Read the model definition and answer for the solid it produces. Units are mm, in the model's axes. A direction names the side the tool comes from. Round coordinates to 2 decimals unless told otherwise and drop trailing zeros. Order: outer loops, then holes, each group sorted by start corner. A loop starts at its lowest first (then second) coordinate and runs counter-clockwise, first axis right, second up. Notation, with made-up numbers: (30, -13.75) - (59, -13.75) arc R16 cw to (59, -6.75) - close; hole circle Ø9 at (22.25, 45.25). An arc over 180 degrees is marked (long way). Answer as a JSON object with one key per item and string values. Group by question number.
Q1. Consider line 1 (Z direction, x = -11, y = 92); line 2 (X direction, y = 104, z = -68.8); line 3 (Z direction, x = 11.5, y = 49). Determine where each line is inside the solid, lowest interval first.
Q2. The mould has two halves that part along Z. Classify faces 4 (the flat face through (-13, -9, 2)), 5 (the flat face through (-19, 52, -40)), 6 (the cylindrical face through (-14.096, -10.369, 3.014)): pulls with the +Z half, pulls with the -Z half, needs draft (parallel to the pull), parting line crosses it, or undercut.
Q3. A cutting plane is placed at D-D on z = -14.5. Determine the outline of the cut face in (x, y).
Q4. Given pin 1 Ø13 at (x, y) = (4.17, 91.16) entering from +Z; pin 2 Ø5 at (x, y) = (-10.92, 111.94) entering from -Z; pin 3 Ø6 at (y, z) = (31, -56) entering from +X; pin 4 Ø2 at (x, z) = (-2.5, -46) entering from -Y, each flat-ended and moving along its own axis, determine where each tip first touches the part or whether it passes through.
Q5. A cutting plane is placed at C-C on y = 28.5. Determine the outline of the cut face in (x, z), and give its area (3 significant figures).
Q6. A cutting plane is placed at A-A on z = -33. Determine the outline of the cut face in (x, y).
Q7. A cutting plane is placed at B-B on y = 0. Determine the outline of the cut face in (x, z).
Q8. A tool of negligible diameter and unlimited length cuts with its end or side. For faces 1 (the flat face through (0, 92, -68)), 2 (the flat face through (0, 12, 0)), 3 (the cylindrical face through (3.305, 120.744, -71.014)), from which of +Z, -Z, +X, -X, +Y, -Y can it reach the whole face along a straight path? Write none if from no direction.
```python
from build123d import *

# Parameters (mm, degrees)
BOSS_EXTRUDE2_DEPTH       = 4
BOSS_EXTRUDE3_START       = 68
BOSS_EXTRUDE3_DEPTH       = 68
BOSS_EXTRUDE4_START       = 4
BOSS_EXTRUDE4_DEPTH       = 4
BOSS_EXTRUDE5_START       = -4
BOSS_EXTRUDE5_DEPTH       = 4
CUT_EXTRUDE1_REACH        = 144.941
CUT_EXTRUDE2_DEPTH        = 143.940547082
BOSS_EXTRUDE7_DEPTH       = 10
BOSS_EXTRUDE7_DEPTH_BACK  = 10
SKETCH10_R                = 2
CUT_EXTRUDE3_DEPTH        = 4
SKETCH11_R                = 18
SKETCH11_R_2              = 16
BOSS_EXTRUDE8_DEPTH       = 4
MIRROR6_COPY_1_SKETCH_R   = 2
MIRROR6_COPY_1_DEPTH      = 4
MIRROR6_COPY_2_SKETCH_R   = 18
MIRROR6_COPY_2_SKETCH_R_2 = 16
MIRROR6_COPY_2_DEPTH      = 4
SKETCH12_R                = 4.000160783
SKETCH12_R_2              = 2
CUT_EXTRUDE5_DEPTH        = 2
MIRROR8_COPY_1_SKETCH_R   = 4.000160783
MIRROR8_COPY_1_SKETCH_R_2 = 2
MIRROR8_COPY_1_DEPTH      = 2
SKETCH13_W                = 4
SKETCH13_H                = 5
BOSS_EXTRUDE9_DEPTH       = 6
SKETCH14_W                = 20
SKETCH14_H                = 5
BOSS_EXTRUDE10_DEPTH      = 4
FILLET1_R                 = 5


with BuildPart() as part:
    # Sketch2 → Boss-Extrude2 (new body)
    with BuildSketch(Plane.XY):
        with BuildLine():
            Line((-16, 0), (-16, 30))
            ThreePointArc((-16, 30), (0, 46), (16, 30))
            Line((16, 30), (16, 0))
            ThreePointArc((16, 0), (0, -16), (-16, 0))
        make_face()
    extrude(amount=BOSS_EXTRUDE2_DEPTH)

    # Sketch3 → Boss-Extrude3 (add)
    with BuildSketch(Plane(origin=(0, 0, 0), x_dir=(-1, 0, 0), z_dir=(0, 0, -1)).offset(BOSS_EXTRUDE3_START)):
        with BuildLine():
            Line((-16, 30), (-16, 26))
            Line((-16, 26), (-12, 30))
            ThreePointArc((-12, 30), (0, 42), (12, 30))
            Line((12, 30), (16, 26))
            Line((16, 26), (16, 30))
            ThreePointArc((16, 30), (0, 46), (-16, 30))
        make_face()
    boss_extrude3 = extrude(amount=-BOSS_EXTRUDE3_DEPTH)

    # Sketch4 → Boss-Extrude4 (add)
    with BuildSketch(Plane(origin=(0, 0, -68), x_dir=(-1, 0, 0), z_dir=(0, 0, -1)).offset(BOSS_EXTRUDE4_START)):
        with BuildLine():
            Line((-16, 30), (-16, 0))
            ThreePointArc((-16, 0), (0, -16), (16, 0))
            Line((16, 0), (16, 30))
            ThreePointArc((16, 30), (0, 46), (-16, 30))
        make_face()
    boss_extrude4 = extrude(amount=-BOSS_EXTRUDE4_DEPTH)

    # Sketch5 → Boss-Extrude5 (add)
    with BuildSketch(Plane.XY.offset(4).offset(BOSS_EXTRUDE5_START)):
        with BuildLine():
            Line((-16, 120), (-16, 30))
            ThreePointArc((-16, 30), (0, 46), (16, 30))
            Line((16, 30), (16, 120))
            Line((16, 120), (-16, 120))
        make_face()
    boss_extrude5 = extrude(amount=BOSS_EXTRUDE5_DEPTH)

    # Mirror3: Boss-Extrude3, Boss-Extrude4 across plane
    add(boss_extrude3.mirror(Plane(origin=(0, 52, 0), x_dir=(0, 0, 1), z_dir=(0, -1, 0))))
    add(boss_extrude4.mirror(Plane(origin=(0, 52, 0), x_dir=(0, 0, 1), z_dir=(0, -1, 0))))

    # Sketch6 → Cut-Extrude1 (cut, up to next)
    with BuildSketch(Plane.XY.offset(4), mode=Mode.PRIVATE) as cut_extrude1_sk1:
        with BuildLine():
            ThreePointArc((-16, 104), (-11.313708499, 115.313708499), (0, 120))
            Line((0, 120), (-16, 120))
            Line((-16, 120), (-16, 104))
        make_face()
    cut_extrude1_tool1 = extrude(cut_extrude1_sk1.sketch, amount=-CUT_EXTRUDE1_REACH, mode=Mode.PRIVATE) & part.part
    # Sketch6 → Cut-Extrude1 (cut, up to next)
    with BuildSketch(Plane.XY.offset(4), mode=Mode.PRIVATE) as cut_extrude1_sk2:
        with BuildLine():
            Line((16, 104), (16, 120))
            Line((16, 120), (0, 120))
            ThreePointArc((0, 120), (11.313708499, 115.313708499), (16, 104))
        make_face()
    cut_extrude1_tool2 = extrude(cut_extrude1_sk2.sketch, amount=-CUT_EXTRUDE1_REACH, mode=Mode.PRIVATE) & part.part
    cut_extrude1_1 = cut_extrude1_tool1.solids().sort_by_distance((-12.426113, 116.426113, 4))[0]
    add(cut_extrude1_1, mode=Mode.SUBTRACT)
    cut_extrude1_2 = cut_extrude1_tool2.solids().sort_by_distance((12.426113, 116.426113, 4))[0]
    add(cut_extrude1_2, mode=Mode.SUBTRACT)
    cut_extrude1 = cut_extrude1_1 + cut_extrude1_2  # Cut-Extrude1 as one shape, for the pattern or mirror that repeats it

    # Mirror4: Boss-Extrude5, Cut-Extrude1 across plane
    add(boss_extrude5.mirror(Plane.XY.offset(-34)))
    add(cut_extrude1.mirror(Plane.XY.offset(-34)), mode=Mode.SUBTRACT)

    # Sketch8 → Cut-Extrude2 (cut, through all)
    with BuildSketch(Plane(origin=(0, 0, -72), x_dir=(-1, 0, 0), z_dir=(0, 0, -1))):
        with BuildLine():
            Line((-16, 74), (-16, 30))
            ThreePointArc((-16, 30), (0, 46), (16, 30))
            Line((16, 30), (16, 74))
            ThreePointArc((16, 74), (0, 58), (-16, 74))
        make_face()
    extrude(amount=-CUT_EXTRUDE2_DEPTH, mode=Mode.SUBTRACT)


with BuildPart() as cut_extrude2_piece_1:
    # of the separate pieces the step leaves, piece 1, a body of its own (cut_extrude2_pieces)
    add(part.part.solids().sort_by_distance((16, 104, 4))[0])



with BuildPart() as cut_extrude2_piece_2:
    # of the separate pieces the step leaves, piece 2, a body of its own (cut_extrude2_pieces)
    add(part.part.solids().sort_by_distance((16, 0, 0))[0])


with BuildPart() as cut_extrude2_piece_1_1:
    add(cut_extrude2_piece_1.part)

    add(cut_extrude2_piece_2.part)  # Boss-Extrude7 merges Cut-Extrude2 piece 2
    # Sketch9 → Boss-Extrude7 (add, two sides: drawn at the far end of the back side and taken through both)
    with BuildSketch(Plane.XY.offset(-34).offset(-BOSS_EXTRUDE7_DEPTH_BACK)):
        with BuildLine():
            Line((-16, 74), (-16, 30))
            ThreePointArc((-16, 30), (0, 46), (16, 30))
            Line((16, 30), (16, 74))
            ThreePointArc((16, 74), (0, 58), (-16, 74))
        make_face()
    extrude(amount=BOSS_EXTRUDE7_DEPTH + BOSS_EXTRUDE7_DEPTH_BACK)

    # Sketch10 → Cut-Extrude3 (cut)
    with BuildSketch(Plane(origin=(0, 0, -72), x_dir=(-1, 0, 0), z_dir=(0, 0, -1))):
        with Locations((-13.5, 0)):
            Circle(SKETCH10_R)
        with Locations((-4.171729424, 12.83926297)):
            Circle(SKETCH10_R)
        with Locations((10.921729424, 7.935100906)):
            Circle(SKETCH10_R)
        with Locations((10.921729424, -7.935100906)):
            Circle(SKETCH10_R)
        with Locations((-4.171729424, -12.83926297)):
            Circle(SKETCH10_R)
    cut_extrude3 = extrude(amount=-CUT_EXTRUDE3_DEPTH, mode=Mode.SUBTRACT)

    # Sketch11 → Boss-Extrude8 (add)
    with BuildSketch(Plane(origin=(0, 0, -72), x_dir=(-1, 0, 0), z_dir=(0, 0, -1))):
        Circle(SKETCH11_R)
        Circle(SKETCH11_R_2, mode=Mode.SUBTRACT)
    boss_extrude8 = extrude(amount=-BOSS_EXTRUDE8_DEPTH)

    # Mirror5: Cut-Extrude3, Boss-Extrude8 across plane
    add(cut_extrude3.mirror(Plane.XY.offset(-34)), mode=Mode.SUBTRACT)
    add(boss_extrude8.mirror(Plane.XY.offset(-34)))

    # Mirror6: Cut-Extrude3, Boss-Extrude8 across plane
    add(cut_extrude3.mirror(Plane(origin=(0, 52, 0), x_dir=(0, 0, 1), z_dir=(0, -1, 0))), mode=Mode.SUBTRACT)
    add(boss_extrude8.mirror(Plane(origin=(0, 52, 0), x_dir=(0, 0, 1), z_dir=(0, -1, 0))))

    # Mirror6 copy 1 sketch → Mirror6 copy 1 (cut)
    with BuildSketch(Plane(origin=(0, 104, 4), x_dir=(-1, 0, 0), z_dir=(0, 0, 1))):
        with Locations((-13.5, 0)):
            Circle(MIRROR6_COPY_1_SKETCH_R)
        with Locations((-4.171729424, 12.83926297)):
            Circle(MIRROR6_COPY_1_SKETCH_R)
        with Locations((10.921729424, 7.935100906)):
            Circle(MIRROR6_COPY_1_SKETCH_R)
        with Locations((10.921729424, -7.935100906)):
            Circle(MIRROR6_COPY_1_SKETCH_R)
        with Locations((-4.171729424, -12.83926297)):
            Circle(MIRROR6_COPY_1_SKETCH_R)
    extrude(amount=-MIRROR6_COPY_1_DEPTH, mode=Mode.SUBTRACT)

    # Mirror6 copy 2 sketch → Mirror6 copy 2 (add)
    with BuildSketch(Plane(origin=(0, 104, 4), x_dir=(-1, 0, 0), z_dir=(0, 0, 1))):
        Circle(MIRROR6_COPY_2_SKETCH_R)
        Circle(MIRROR6_COPY_2_SKETCH_R_2, mode=Mode.SUBTRACT)
    extrude(amount=-MIRROR6_COPY_2_DEPTH)

    # Sketch12 → Cut-Extrude5 (cut)
    # profile 1 of 5: a face of its own
    with BuildSketch(Plane.XY.offset(4)):
        with Locations((-10.921729424, 7.935100906)):
            Circle(SKETCH12_R)
        with Locations((-10.921729424, 7.935100906)):
            Circle(SKETCH12_R_2, mode=Mode.SUBTRACT)
    # profile 2 of 5: a face of its own
    with BuildSketch(Plane.XY.offset(4)):
        with Locations((4.171729424, 12.83926297)):
            Circle(SKETCH12_R)
        with Locations((4.171729424, 12.83926297)):
            Circle(SKETCH12_R_2, mode=Mode.SUBTRACT)
    # profile 3 of 5: a face of its own
    with BuildSketch(Plane.XY.offset(4)):
        with Locations((13.5, 0)):
            Circle(SKETCH12_R)
        with Locations((13.5, 0)):
            Circle(SKETCH12_R_2, mode=Mode.SUBTRACT)
    # profile 4 of 5: a face of its own
    with BuildSketch(Plane.XY.offset(4)):
        with Locations((4.171729424, -12.83926297)):
            Circle(SKETCH12_R)
        with Locations((4.171729424, -12.83926297)):
            Circle(SKETCH12_R_2, mode=Mode.SUBTRACT)
    # profile 5 of 5: a face of its own
    with BuildSketch(Plane.XY.offset(4)):
        with Locations((-10.921729424, -7.935100906)):
            Circle(SKETCH12_R)
        with Locations((-10.921729424, -7.935100906)):
            Circle(SKETCH12_R_2, mode=Mode.SUBTRACT)
    cut_extrude5 = extrude(amount=-CUT_EXTRUDE5_DEPTH, mode=Mode.SUBTRACT)

    # Mirror7: Cut-Extrude5 across plane
    add(cut_extrude5.mirror(Plane.XY.offset(-34)), mode=Mode.SUBTRACT)

    # Mirror8: Cut-Extrude5 across plane
    add(cut_extrude5.mirror(Plane(origin=(0, 52, 0), x_dir=(0, 0, 1), z_dir=(0, -1, 0))), mode=Mode.SUBTRACT)

    # Mirror8 copy 1 sketch → Mirror8 copy 1 (cut)
    # profile 1 of 5: a face of its own
    with BuildSketch(Plane(origin=(0, 104, -72), x_dir=(1, 0, 0), z_dir=(0, 0, -1))):
        with Locations((-10.921729424, 7.935100906)):
            Circle(MIRROR8_COPY_1_SKETCH_R)
        with Locations((-10.921729424, 7.935100906)):
            Circle(MIRROR8_COPY_1_SKETCH_R_2, mode=Mode.SUBTRACT)
    # profile 2 of 5: a face of its own
    with BuildSketch(Plane(origin=(0, 104, -72), x_dir=(1, 0, 0), z_dir=(0, 0, -1))):
        with Locations((4.171729424, 12.83926297)):
            Circle(MIRROR8_COPY_1_SKETCH_R)
        with Locations((4.171729424, 12.83926297)):
            Circle(MIRROR8_COPY_1_SKETCH_R_2, mode=Mode.SUBTRACT)
    # profile 3 of 5: a face of its own
    with BuildSketch(Plane(origin=(0, 104, -72), x_dir=(1, 0, 0), z_dir=(0, 0, -1))):
        with Locations((13.5, 0)):
            Circle(MIRROR8_COPY_1_SKETCH_R)
        with Locations((13.5, 0)):
            Circle(MIRROR8_COPY_1_SKETCH_R_2, mode=Mode.SUBTRACT)
    # profile 4 of 5: a face of its own
    with BuildSketch(Plane(origin=(0, 104, -72), x_dir=(1, 0, 0), z_dir=(0, 0, -1))):
        with Locations((4.171729424, -12.83926297)):
            Circle(MIRROR8_COPY_1_SKETCH_R)
        with Locations((4.171729424, -12.83926297)):
            Circle(MIRROR8_COPY_1_SKETCH_R_2, mode=Mode.SUBTRACT)
    # profile 5 of 5: a face of its own
    with BuildSketch(Plane(origin=(0, 104, -72), x_dir=(1, 0, 0), z_dir=(0, 0, -1))):
        with Locations((-10.921729424, -7.935100906)):
            Circle(MIRROR8_COPY_1_SKETCH_R)
        with Locations((-10.921729424, -7.935100906)):
            Circle(MIRROR8_COPY_1_SKETCH_R_2, mode=Mode.SUBTRACT)
    extrude(amount=-MIRROR8_COPY_1_DEPTH, mode=Mode.SUBTRACT)

    # Sketch13 → Boss-Extrude9 (add)
    with BuildSketch(Plane.ZY.offset(16)):
        with Locations((-42, 52)):
            Rectangle(SKETCH13_W, SKETCH13_H)
        with Locations((-26, 52)):
            Rectangle(SKETCH13_W, SKETCH13_H)
    extrude(amount=BOSS_EXTRUDE9_DEPTH)

    # Sketch14 → Boss-Extrude10 (add)
    with BuildSketch(Plane.ZY.offset(22)):
        with Locations((-34, 52)):
            Rectangle(SKETCH14_W, SKETCH14_H)
    extrude(amount=BOSS_EXTRUDE10_DEPTH)

    # Fillet1
    fillet1_edges = [cut_extrude2_piece_1_1.edges().sort_by_distance(p)[0] for p in [
        (-26, 52, -44),
        (-26, 52, -24),
    ]]
    fillet(fillet1_edges, radius=FILLET1_R)


solid = cut_extrude2_piece_1_1.part
```
Result set:
{
 "1": {"line 1": "z = -72 to -68, 0 to 4", "line 2": "x = -18 to 11.5, 15.5 to 18", "line 3": "z = -44 to -24"},
 "2": {"face 4": "pulls with the +Z half", "face 5": "undercut", "face 6": "needs draft"},
 "3": {"outline": "(-16, 26) - (-12, 30) arc R12 cw to (12, 30) - (16, 26) - (16, 30) arc R16 ccw to (-16, 30) - close; (-16, 74) arc R16 ccw to (16, 74) - (16, 78) - (12, 74) arc R12 cw to (-12, 74) - (-16, 78) - close"},
 "4": {"pin 1": "stops at z = 4", "pin 2": "stops at z = -70", "pin 3": "stops at x = 16", "pin 4": "stops at y = 41.48"},
 "5": {"outline": "(-16, -72) - (16, -72) - (16, 4) - (-16, 4) - close; hole (-13.5, -68) - (13.5, -68) - (13.5, 0) - (-13.5, 0) - close", "area": "596 mm²"},
 "6": {"outline": "(-26, 49.5) - (-22, 49.5) - (-22, 54.5) - (-26, 54.5) - close; (-16, 26) - (-12, 30) arc R12 cw to (12, 30) - (16, 26) - (16, 78) - (12, 74) arc R12 cw to (-12, 74) - (-16, 78) - close"},
 "7": {"outline": "(-18, -72) - (9.5, -72) - (9.5, -70) - (11.5, -70) - (11.5, -68) - (-18, -68) - close; (-18, 0) - (11.5, 0) - (11.5, 2) - (9.5, 2) - (9.5, 4) - (-18, 4) - close; (15.5, -70) - (17.5, -70) - (17.5, -72) - (18, -72) - (18, -68) - (15.5, -68) - close; (15.5, 0) - (18, 0) - (18, 4) - (17.5, 4) - (17.5, 2) - (15.5, 2) - close"},
 "8": {"face 1": "+Y", "face 2": "-Y", "face 3": "-Z"}
}
